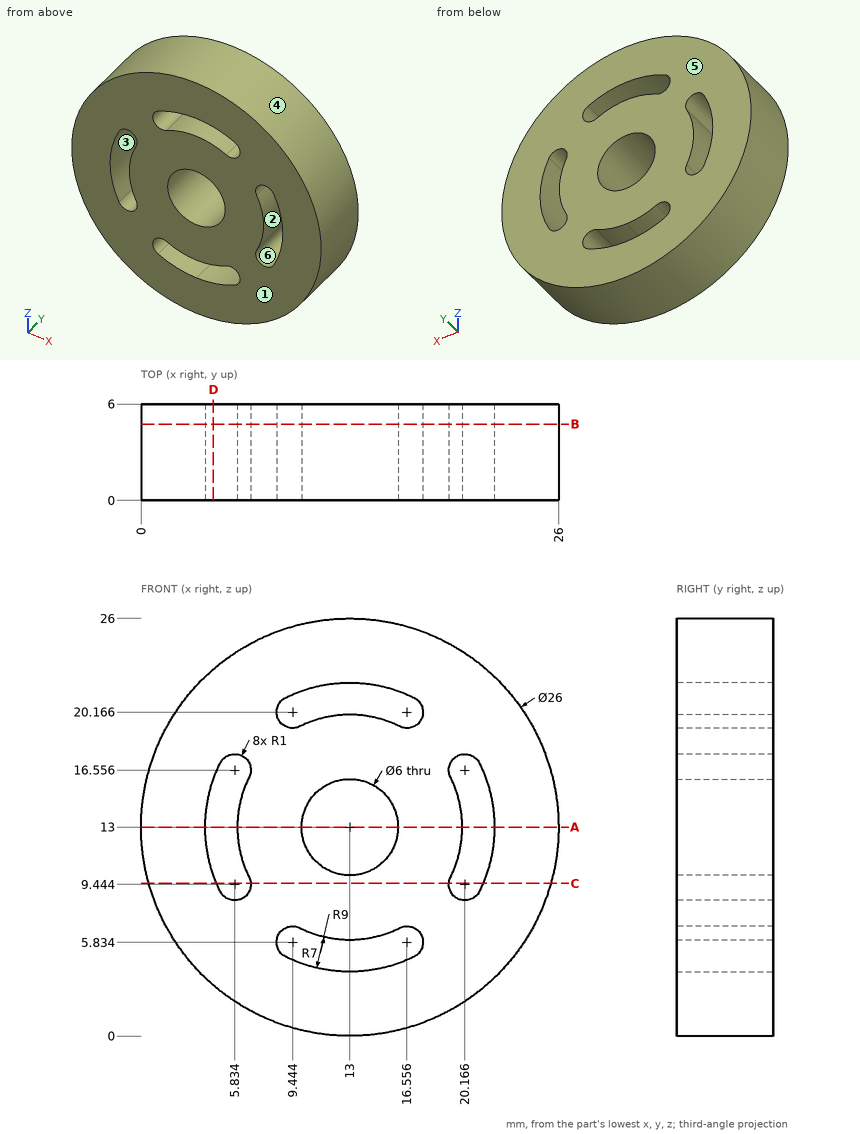
Geometry check sheet. Reference: drawing and pictorial views, mm from the part's lowest x, y, z. A direction names the side the tool comes from. Round coordinates to 2 decimals unless told otherwise and drop trailing zeros. Loops run counter-clockwise (first coordinate to the right, second up) from the corner with the lowest first, then second, coordinate; pieces in that order, holes last.
1. Set-up check for the marked faces 1 and 2: record each of +Z, -Z, +X, -X, +Y, -Y from which the full face is reachable in a straight line by a thin tool's end or side.
2. Gauge pin test, flat ends, axial feed: pin 1 Ø8 at (x, z) = (13, 13) entering from +Y; pin 2 Ø1 at (x, y) = (7.5, 5.5) entering from +Z; pin 3 Ø2 at (x, y) = (18, 4.5) entering from +Z. Record the tip position at first contact, or that the pin passes through.
3. Sectioned sample at D-D on x = 4.5. Record the boundary of the cut face in (y, z).
4. Sectioned sample at B-B on y = 4.75. Record the boundary of the cut face in (x, z) (1 decimal).
5. Mould release check, pull along X, two halves, no side actions. Record for the marked faces 3, 4, 5 and 6: released by +X, released by -X, zero draft, split by the parting line, or undercut.
6. Sectioned sample at A-A on z = 13. Record the boundary of the cut face in (x, y).
7. Scan lines: probe 1 along X at (y, z) = (3.45, 13); probe 2 along Z at (x, y) = (10.25, 5.5) (1 decimal); probe 3 along X at (y, z) = (2.15, 11.75). Record each from-to range of solid material in increasing order.
8. Sectioned sample at C-C on z = 9.5. Record the boundary of the cut face in (x, y).
Recorded:
1. face 1: +Z, -Z, +X, -X, -Y
1. face 2: +Y, -Y
2. pin 1: stops at y = 6
2. pin 2: stops at z = 25
2. pin 3: stops at z = 25.37
3. outline: (0, 3.16) - (6, 3.16) - (6, 10.04) - (0, 10.04) - close; (0, 15.96) - (6, 15.96) - (6, 22.84) - (0, 22.84) - close
4. outline: circle Ø26 at (13, 13); hole (4.9, 9) arc R1 ccw to (6.7, 9.9) arc R7 cw to (6.7, 16.1) arc R1 ccw to (4.9, 17) arc R9 ccw to start; hole (9, 4.9) arc R9 ccw to (17, 4.9) arc R1 ccw to (16.1, 6.7) arc R7 cw to (9.9, 6.7) arc R1 ccw to start; hole (9, 21.1) arc R1 ccw to (9.9, 19.3) arc R7 cw to (16.1, 19.3) arc R1 ccw to (17, 21.1) arc R9 ccw to start; hole circle Ø6 at (13, 13); hole (19.3, 9.9) arc R1 ccw to (21.1, 9) arc R9 ccw to (21.1, 17) arc R1 ccw to (19.3, 16.1) arc R7 cw to start
5. face 3: undercut
5. face 4: split by the parting line
5. face 5: zero draft
5. face 6: undercut
6. outline: (0, 0) - (4, 0) - (4, 6) - (0, 6) - close; (6, 0) - (10, 0) - (10, 6) - (6, 6) - close; (16, 0) - (20, 0) - (20, 6) - (16, 6) - close; (22, 0) - (26, 0) - (26, 6) - (22, 6) - close
7. probe 1: x = 0 to 4, 6 to 10, 16 to 20, 22 to 26
7. probe 2: z = 0.3 to 4.4, 6.6 to 11.8, 14.2 to 19.4, 21.6 to 25.7
7. probe 3: x = 0.06 to 4.09, 6.11 to 10.27, 15.73 to 19.89, 21.91 to 25.94
8. outline: (0.48, 0) - (4.71, 0) - (4.71, 6) - (0.48, 6) - close; (6.83, 0) - (19.17, 0) - (19.17, 6) - (6.83, 6) - close; (21.29, 0) - (25.52, 0) - (25.52, 6) - (21.29, 6) - close
